The listing builds one solid part. Answer for the finished solid, in the listing's coordinates (mm). A direction names the side the tool comes from. Coordinates: 2 decimals unless noted, no trailing zeros. Write each loop counter-clockwise with the first axis right and the second up, starting at its lowest first coordinate (ties: lowest second). Pieces come first, ordered by that corner, then holes.
from build123d import *

# Parameters (mm, degrees)
F1_DEPTH  = 2
F2_R      = 2.75
F3_DEPTH  = 13
F6_DEPTH  = 3
F8_W      = 20
F8_H      = 2
F11_DEPTH = 1
F13_DEPTH = 5
F14_R     = 2


with BuildPart() as f1:
    # F0 (on Top) → F1 (new body)
    with BuildSketch(Plane.XY):
        with BuildLine():
            ThreePointArc((7.2, 20), (0, 27.2), (-7.2, 20))
            Line((-7.2, 20), (-7.2, -20))
            ThreePointArc((-7.2, -20), (0, -27.2), (7.2, -20))
            Line((7.2, -20), (7.2, 20))
        make_face()
    extrude(amount=F1_DEPTH)

    # F2 (on face) → F3 (join)
    with BuildSketch(Plane.XY.offset(2)):
        with Locations((0, 20)):
            Circle(F2_R)
        with Locations((0, -20)):
            Circle(F2_R)
    extrude(amount=F3_DEPTH)



with BuildPart() as f6:
    # F5 (on offset) → F6 (new body)
    with BuildSketch(Plane.XZ.offset(28.5)):
        with BuildLine():
            Line((20, 0), (32.75, 0))
            Line((32.75, 0), (32.75, 3))
            Line((32.75, 3), (28.75, 3))
            ThreePointArc((28.75, 3), (24.5, 7.25), (28.75, 11.5))
            Line((28.75, 11.5), (32.75, 11.5))
            Line((32.75, 11.5), (32.75, 13.5))
            Line((32.75, 13.5), (20, 13.5))
            Line((20, 13.5), (20, 0))
        make_face()
    extrude(amount=-F6_DEPTH)


with BuildPart() as f1_1:
    add(f1.part)

    add(f6.part)  # F9 merges F6
    # F7 (on face) → F9 section 0
    with BuildSketch(Plane(origin=(20, 0, 0), x_dir=(0, -1, 0), z_dir=(-1, 0, 0))):
        Polygon((16, 0), (28.5, 0), (28.5, 13.5), (25.5, 13.5), align=None)
    # F8 (on face) → F9 section 1
    with BuildSketch(Plane.YZ.offset(7.2)):
        with Locations((-1, 1)):
            Rectangle(F8_W, F8_H)
    loft()

    # F10 (on face) → F11 (join)
    with BuildSketch(Plane(origin=(0, 0, 0), x_dir=(1, 0, 0), z_dir=(0, 0, -1))):
        Polygon((20, 16), (32.75, 25.5), (20, 25.5), align=None)
    extrude(amount=-F11_DEPTH)

    # F12 (on face) → F13 (join)
    with BuildSketch(Plane.XY.offset(2)):
        with BuildLine():
            ThreePointArc((7.2, 20), (0, 27.2), (-7.2, 20))
            ThreePointArc((-7.2, 20), (0, 12.8), (7.2, 20))
        make_face()
        with BuildLine():
            ThreePointArc((-7.2, -20), (0, -27.2), (7.2, -20))
            ThreePointArc((7.2, -20), (0, -12.8), (-7.2, -20))
        make_face()
    extrude(amount=F13_DEPTH)

    # F14
    f14_edges = [f1_1.edges().sort_by_distance(p)[0] for p in [
        (-2.75, 20, 15),
        (-2.75, -20, 15),
    ]]
    fillet(f14_edges, radius=F14_R)


solid = f1_1.part
Q1. The part is cut by section C-C, the plane y = 11. Write down the section's boundary in (x, z).
Answers below:
outline: (-7.2, 0) - (7.2, 0) - (7.2, 2) - (-7.2, 2) - close
Q2. The part is cut by section B-B, the plane z = 5.75. State how many separate pieces and enclosed holes the cut face has, then the cut area to 3 significant figures.
Answers below:
separate pieces: 3
enclosed holes: 0
area: 438 mm2
Q3. Determine the mould class of faces 1 (the face through (0, -20, 15)), 2 (the face through (-0.358, -17.273, 9.958)), 3 (the face through (23, -25.5, 7)) for opening direction Y: released by +Y, released by -Y, zero draft, split by the parting line, or undercut.
Answers below:
face 1: zero draft
face 2: undercut
face 3: released by +Y
Q4. The part is cut by section A-A, the plane x = 30. Write down the section's boundary in (y, z).
Answers below:
outline: (-28.5, 0) - (-23.45, 0) - (-23.45, 1) - (-25.5, 1) - (-25.5, 3) - (-28.5, 3) - close; (-28.5, 11.5) - (-25.5, 11.5) - (-25.5, 13.5) - (-28.5, 13.5) - close
Q5. Find the intervals of material crossed by probe 1 along Z at (x, y) = (5, -5.5); probe 2 along Y at (x, z) = (24, 1.5); probe 3 along Y at (x, z) = (-2, 6.25), in increasing order.
Answers below:
probe 1: z = 0 to 2
probe 2: y = -28.5 to -25.5
probe 3: y = -26.92 to -13.08, 13.08 to 26.92
Q6. Given pin 1 (6 mm diameter, centred on x = 27.5, z = 6.5, fed in from +Y); pin 2 (5 mm diameter, centred on x = 9.5, y = -19.5, fed in from +Z); pin 3 (16 mm diameter, centred on x = -2.5, y = 3.5, fed in from +Z); pin 4 (5 mm diameter, centred on y = 10, z = 5.5, fed in from +X), each flat-ended and moving along its own axis, determine where each tip first touches the part or whether it passes through.
Answers below:
pin 1: stops at y = -25.5
pin 2: stops at z = 7
pin 3: stops at z = 2
pin 4: passes through
Q7. Which of the six approach directions +Z, -Z, +X, -X, +Y, -Y give full straight-line access (tool end or side, diameter ignored) to faces 4 (the face through (0, -23, 7)), 5 (the face through (7.2, 14, 1)), 6 (the face through (31, -27, 11.5))?
Answers below:
face 4: +Z
face 5: +Z, -Z, +X, +Y
face 6: +X, +Y, -Y
